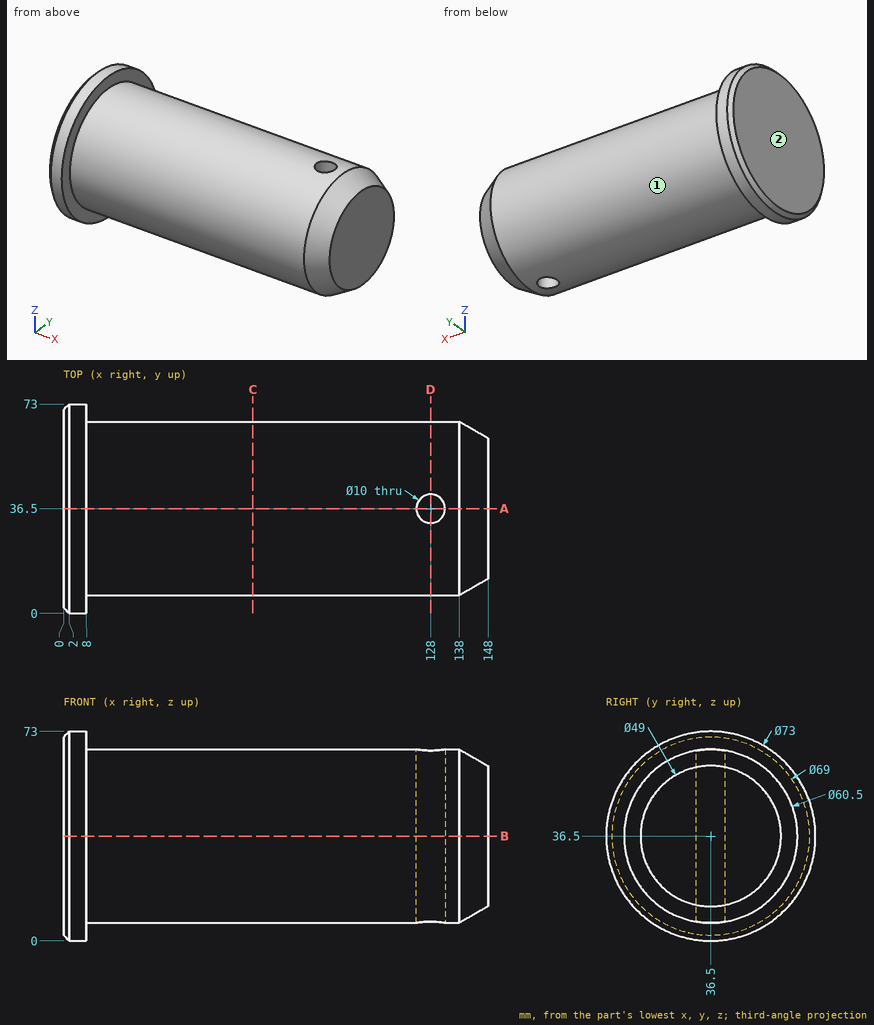
Drawing for the job (mm, zero at the part's lowest x, y, z). A direction names the side the tool comes from. Round coordinates to 2 decimals unless told otherwise and drop trailing zeros. Order: outer loops, then holes, each group sorted by start corner. A loop starts at its lowest first (then second) coordinate and runs counter-clockwise, first axis right, second up.
Item 1: Saw through at C-C on x = 66. Write the cut outline in (y, z), then the cut area to 3 significant figures.
Item 2: Tool access for the marked faces 1 and 2: list every direction of +Z, -Z, +X, -X, +Y, -Y with a clear straight run to the whole face (end or side of a thin tool).
Item 3: Saw through at B-B on z = 36.5. Write the cut outline in (x, y).
Item 4: Saw through at A-A on y = 36.5. Write the cut outline in (x, z).
Item 5: Pin check, flat tips, straight feed: pin 1 (1 mm diameter, centred on x = 121, y = 54.5, fed in from -Z); pin 2 (2 mm diameter, centred on x = 29.5, z = 45, fed in from -Y); pin 3 (16 mm diameter, centred on x = 128, y = 36.5, fed in from +Z). Stop position of each tip, or through.
Item 6: Saw through at D-D on x = 128. Write the cut outline in (y, z), then the cut area to 3 significant figures.
Item 7: Probe line 1 along X through (y, z) = (36, 20); line 2 along Y through (x, z) = (41, 37); line 3 along Y through (x, z) = (128, 25.5). List the from-to ranges inside material, lowest first.
Reported:
1. outline: circle Ø60.5 at (36.5, 36.5)
1. area: 2,870 mm2
2. face 1: +X
2. face 2: +Z, -Z, -X, +Y, -Y
3. outline: (0, 2) - (2, 0) - (8, 0) - (8, 6.25) - (138, 6.25) - (148, 12) - (148, 61) - (138, 66.75) - (8, 66.75) - (8, 73) - (2, 73) - (0, 71) - close; hole circle Ø10 at (128, 36.5)
4. outline: (0, 2) - (2, 0) - (8, 0) - (8, 6.25) - (123, 6.25) - (123, 66.75) - (8, 66.75) - (8, 73) - (2, 73) - (0, 71) - close; (133, 6.25) - (138, 6.25) - (148, 12) - (148, 61) - (138, 66.75) - (133, 66.75) - close
5. pin 1: stops at z = 11.83
5. pin 2: stops at y = 7.19
5. pin 3: stops at z = 66.75
6. outline: (31.5, 6.67) - (31.5, 66.33) arc R30.25 ccw to start; (41.5, 6.67) arc R30.25 ccw to (41.5, 66.33) - close
6. area: 2,270 mm2
7. line 1: x = 0 to 123.03, 132.97 to 148
7. line 2: y = 6.25 to 66.75
7. line 3: y = 8.32 to 31.5, 41.5 to 64.68
